```python
from build123d import *

# Parameters (mm, degrees)
SKETCH1_R           = 1.4224
BOSS_EXTRUDE1_DEPTH = 9.525
SKETCH2_R           = 2.7051
BOSS_EXTRUDE2_DEPTH = 1.4986
FILLET1_R           = 1.016
CUT_EXTRUDE1_DEPTH  = 2.38125


with BuildPart() as part:
    # Sketch1 → Boss-Extrude1 (new body)
    with BuildSketch(Plane(origin=(0, 0, 0), x_dir=(1, 0, 0), z_dir=(0, 1, 0))):
        Circle(SKETCH1_R)
    extrude(amount=BOSS_EXTRUDE1_DEPTH)

    # Sketch2 → Boss-Extrude2 (add)
    with BuildSketch(Plane(origin=(0, 9.525, 0), x_dir=(1, 0, 0), z_dir=(0, 1, 0))):
        Circle(SKETCH2_R)
    extrude(amount=BOSS_EXTRUDE2_DEPTH)

    # Fillet1
    fillet1_edges = [part.edges().sort_by_distance(p)[0] for p in [
        (-2.7051, 11.0236, 0),
    ]]
    fillet(fillet1_edges, radius=FILLET1_R)

    # Sketch3 → Cut-Extrude1 (cut)
    with BuildSketch(Plane(origin=(0, 11.0236, 0), x_dir=(1, 0, 0), z_dir=(0, 1, 0))):
        Polygon((0, 0.916543552), (-0.79375, 0.458271776), (-0.79375, -0.458271776), (0, -0.916543552), (0.79375, -0.458271776), (0.79375, 0.458271776), align=None)
    extrude(amount=-CUT_EXTRUDE1_DEPTH, mode=Mode.SUBTRACT)


solid = part.part
```
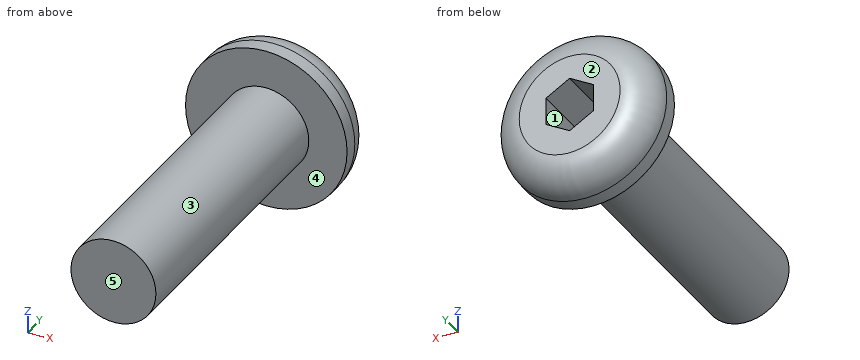
Verification items for the finished model (mm, model axes). Face numbers are marked on the shaded views. A direction names the side the tool comes from. Give positions to 0.01 mm unless a question says otherwise; leave off trailing zeros. Order: outer loops, then holes, each group sorted by start corner. A loop starts at its lowest first (then second) coordinate and runs counter-clockwise, first axis right, second up. Notation, with made-up numbers: (31.25, 45) - (68.25, 45) arc R15 ccw to (68.25, 71) - close; hole circle Ø3 at (1, 80). An arc over 180 degrees is marked (long way). Answer as CSV lines item,"result". Start each with the question number.
Item 1: Gauge pin test, flat ends, axial feed: pin 1 (2 mm diameter, centred on y = 3, z = -0.5, fed in from +X); pin 2 (3 mm diameter, centred on x = -1.5, y = 3, fed in from -Z); pin 3 (0.5 mm diameter, centred on x = 0, z = 0, fed in from +Y). Record the tip position at first contact, or that the pin passes through.
Item 2: Access from +Z, -Z, +X, -X, +Y, -Y to the whole of each face (thin tool, end or side, straight path). Record for the marked faces 4 and 5.
Item 3: Section check A-A, the plane y = 9.75. Record the boundary of the cut face in (x, z), plus the area to 3 significant figures.
Item 4: Material ranges on L1, parallel to Y at x = 0.8, z = 1.35 (3 decimals); L2, parallel to X at y = 10, z = -0.1; L3, parallel to X at y = 6.25, z = 0.75, recorded low to high.
Item 5: Section check C-C, the plane y = 2.75. Record the boundary of the cut face in (x, z), plus the area to 3 significant figures.
Item 6: Mould release check, pull along X, two halves, no side actions. Record for the marked faces 1, 2 and 3: released by +X, released by -X, zero draft, split by the parting line, or undercut.
Item 7: Section check B-B, the plane z = 0. Record the boundary of the cut face in (x, y) (3 decimals).
Filled in:
1,pin 1,"x = 1.42"
1,pin 2,"z = -1.42"
1,pin 3,"y = 8.64"
2,face 4,"-Y"
2,face 5,"+Z, -Z, +X, -X, -Y"
3,outline,"circle Ø5.41 at (0, 0); hole (-0.79, -0.46) - (0, -0.92) - (0.79, -0.46) - (0.79, 0.46) - (0, 0.92) - (-0.79, 0.46) - close"
3,area,"20.8 mm^2"
4,L1,"9.525 to 11.024"
4,L2,"-2.7 to -0.79, 0.79 to 2.7"
4,L3,"-1.21 to 1.21"
5,outline,"circle Ø2.84 at (0, 0)"
5,area,"6.36 mm^2"
6,face 1,"undercut"
6,face 2,"zero draft"
6,face 3,"split by the parting line"
7,outline,"(-2.705, 9.525) - (-1.422, 9.525) - (-1.422, 0) - (1.422, 0) - (1.422, 9.525) - (2.705, 9.525) - (2.705, 10.008) arc R1.016 ccw to (1.689, 11.024) - (0.794, 11.024) - (0.794, 8.642) - (-0.794, 8.642) - (-0.794, 11.024) - (-1.689, 11.024) arc R1.016 ccw to (-2.705, 10.008) - close"
